```python
from build123d import *

# Parameters (mm, degrees)
SKETCH1_W           = 50.8
SKETCH1_H           = 25.4
BOSS_EXTRUDE1_DEPTH = 254
SHELL1_T            = -3.175
SKETCH2_R           = 2.38125
CUT_EXTRUDE1_DEPTH  = 257.527425434
SKETCH3_R           = 2.38125
CUT_EXTRUDE2_DEPTH  = 257.527425434


with BuildPart() as part:
    # Sketch1 → Boss-Extrude1 (new, symmetric)
    with BuildSketch(Plane(origin=(0, 0, 0), x_dir=(1, 0, 0), z_dir=(0, 1, 0))):
        Rectangle(SKETCH1_W, SKETCH1_H)
    extrude(amount=BOSS_EXTRUDE1_DEPTH, both=True)

    # Shell1
    shell1_openings = [part.faces().sort_by_distance(p)[0] for p in [
        (0, 254, 0),
        (0, -254, 0),
    ]]
    offset(amount=SHELL1_T, openings=shell1_openings, kind=Kind.INTERSECTION)

    # Sketch2 → Cut-Extrude1 (cut, through all)
    with BuildSketch(Plane(origin=(0, 0, -12.7), x_dir=(-1, 0, 0), z_dir=(0, 0, -1))):
        with Locations((12.7, -12.7)):
            Circle(SKETCH2_R)
        with Locations((12.7, 12.7)):
            Circle(SKETCH2_R)
    extrude(amount=-CUT_EXTRUDE1_DEPTH, mode=Mode.SUBTRACT)

    # Sketch3 → Cut-Extrude2 (cut, through all)
    with BuildSketch(Plane(origin=(0, 0, -12.7), x_dir=(-1, 0, 0), z_dir=(0, 0, -1))):
        with Locations((0, -241.3)):
            Circle(SKETCH3_R)
        with Locations((12.7, -241.3)):
            Circle(SKETCH3_R)
        with Locations((-12.7, -241.3)):
            Circle(SKETCH3_R)
        with Locations((-12.7, 241.3)):
            Circle(SKETCH3_R)
        with Locations((12.7, 241.3)):
            Circle(SKETCH3_R)
        with Locations((0, 241.3)):
            Circle(SKETCH3_R)
    extrude(amount=-CUT_EXTRUDE2_DEPTH, mode=Mode.SUBTRACT)


solid = part.part
```
Part model, mm, in its own coordinate system. A direction names the side the tool comes from. Round coordinates to 2 decimals unless told otherwise and drop trailing zeros. Loops run counter-clockwise (first coordinate to the right, second up) from the corner with the lowest first, then second, coordinate; pieces in that order, holes last. Notation, with made-up numbers: (-5.5, 22) -> (18.5, 22) arc R26 ccw to (18.5, 39) -> close; hole circle Ø6 at (-29, -17.75). An arc over 180 degrees is marked (long way). Use a Markdown table: item, result.
1) Tool access for faces 4 (the flat face through (0, 4, -12.7)), 5 (the flat face through (22.225, 4, 0)): list every direction of +Z, -Z, +X, -X, +Y, -Y with a clear straight run to the whole face (end or side of a thin tool).
The answers:
| item | result |
|---|---|
| face 4 | -Z, +X, -X, +Y, -Y |
| face 5 | +Y, -Y |
2) Probe line 1 (Y direction, x = -12.7, z = 10.3); line 2 (Z direction, x = 5, y = -159.5) (3 decimals); line 3 (X direction, y = -40, z = -3.75) (3 decimals). List the from-to ranges inside material, lowest first. Write a range as [from, to].
The answers:
| item | result |
|---|---|
| line 1 | y = [-254, -243.68], [-238.92, -15.08], [-10.32, 10.32], [15.08, 238.92], [243.68, 254] |
| line 2 | z = [-12.7, -9.525], [9.525, 12.7] |
| line 3 | x = [-25.4, -22.225], [22.225, 25.4] |
3) Cut at A-A, the plane z = -5.5. List the corners of the cut face in (x, y) (3 decimals).
The answers:
| item | result |
|---|---|
| outline | (-25.4, -254) -> (-22.225, -254) -> (-22.225, 254) -> (-25.4, 254) -> close; (22.225, -254) -> (25.4, -254) -> (25.4, 254) -> (22.225, 254) -> close |
4) Pull direction X, two halves, no side cores. Call faces 1 (the flat face through (-25.4, 4, 0)), 2 (the flat face through (0, 4, 9.525)), 3 (the flat face through (25.4, 4, 0)): pulls with the +X half, pulls with the -X half, needs draft (parallel to the pull), parting line crosses it, or undercut.
The answers:
| item | result |
|---|---|
| face 1 | pulls with the -X half |
| face 2 | undercut |
| face 3 | pulls with the +X half |
5) Cut at B-B, the plane y = -156. List the corners of the cut face in (x, z) (3 decimals).
The answers:
| item | result |
|---|---|
| outline | (-25.4, -12.7) -> (25.4, -12.7) -> (25.4, 12.7) -> (-25.4, 12.7) -> close; hole (-22.225, -9.525) -> (22.225, -9.525) -> (22.225, 9.525) -> (-22.225, 9.525) -> close |
